```python
from build123d import *

# Parameters (mm, degrees)
EXTRUDE_THIN2_DEPTH = 25
SKETCH4_R           = 2.5
CUT_EXTRUDE1_DEPTH  = 0.3


with BuildPart() as part:
    # Sketch1 → Revolve1 (revolve)
    with BuildSketch(Plane.XY):
        Polygon((3.1, 16), (3.1, -16), (20, -16), (20, -12.5), (17, -12.5), (17, 12.5), (20, 12.5), (20, 16), align=None)
    revolve(axis=Axis((0, -1363.747655385, 0), (0, 1, 0)))

    # Sketch2 → Extrude-Thin2 (add)
    with BuildSketch(Plane(origin=(0, -12.5, 0), x_dir=(1, 0, 0), z_dir=(0, 1, 0))):
        with BuildLine():
            ThreePointArc((0, 17), (-17, 0), (0, -17))
            Line((0, -17), (89.2, -17))
            ThreePointArc((89.2, -17), (101.274072829, -7.735238064), (95.45, 6.325317547))
            Line((95.45, 6.325317547), (72.5003268, 19.575317547))
            Line((72.5003268, 19.575317547), (72.6503268, 19.835125168))
            Line((72.6503268, 19.835125168), (95.6, 6.585125168))
            ThreePointArc((95.6, 6.585125168), (101.563850577, -7.812883777), (89.2, -17.3))
            Line((89.2, -17.3), (0, -17.3))
            ThreePointArc((0, -17.3), (-17.3, 0), (0, 17.3))
            Line((0, 17.3), (0, 17))
        make_face()
    extrude(amount=EXTRUDE_THIN2_DEPTH)

    # Sketch4 → Cut-Extrude1 (cut)
    with BuildSketch(Plane(origin=(26.751442841, 0, -46.334858177), x_dir=(-0.866025404, 0, -0.5), z_dir=(0.5, 0, -0.866025404))):
        with Locations((-58.499466018, -7.5)):
            Circle(SKETCH4_R)
        with Locations((-58.499466018, 7.5)):
            Circle(SKETCH4_R)
    extrude(amount=-CUT_EXTRUDE1_DEPTH, mode=Mode.SUBTRACT)


solid = part.part
```
Input: part model. Units: mm. Frame: model coordinates. A direction names the side the tool comes from. Coordinates: 2 decimals unless noted, no trailing zeros. Order: outer loops, then holes, each group sorted by start corner. A loop starts at its lowest first (then second) coordinate and runs counter-clockwise, first axis right, second up. Notation, with made-up numbers: (-20, -7.5) - (12, -7.5) arc R28 cw to (12, 12.5) - close; hole circle Ø1 at (19.25, 57). An arc over 180 degrees is marked (long way). Return JSON: item names as keys, results as strings.
Q1. Cut plane B-B (z = -9.5). Return loops of the section in (x, y).
The answers:
{"outline": "(-17.6, -16) - (17.6, -16) - (17.6, -12.5) - (14.1, -12.5) - (14.1, 12.5) - (17.6, 12.5) - (17.6, 16) - (-17.6, 16) - (-17.6, 12.5) - (-14.46, 12.5) - (-14.46, -12.5) - (-17.6, -12.5) - close; (89.95, -12.5) - (90.55, -12.5) - (90.55, 12.5) - (89.95, 12.5) - close"}
Q2. Ray query, probe 1 along Y at (x, z) = (-6, 16.5); probe 2 along X at (y, z) = (1, 0); probe 3 along X at (y, z) = (4, 14). Return the intervals inside material, ascending.
The answers:
{"probe 1": "y = -16 to -12.5, 12.5 to 16", "probe 2": "x = -17.3 to -3.1, 3.1 to 17, 100.86 to 101.18", "probe 3": "x = -10.16 to 9.64, 97.32 to 97.78"}
Q3. Cut plane D-D (z = 14.5). Return loops of the section in (x, y).
The answers:
{"outline": "(-13.77, -16) - (13.77, -16) - (13.77, -12.5) - (8.87, -12.5) - (8.87, 12.5) - (13.77, 12.5) - (13.77, 16) - (-13.77, 16) - (-13.77, 12.5) - (-9.44, 12.5) - (-9.44, -12.5) - (-13.77, -12.5) - close; (96.7, -12.5) - (97.19, -12.5) - (97.19, 12.5) - (96.7, 12.5) - close"}
Q4. First-contact query: pin 1 (2 mm diameter, centred on x = -1, y = 0.5, fed in from +Z); pin 2 (1 mm diameter, centred on x = 11, y = 6.5, fed in from -Z); pin 3 (4 mm diameter, centred on x = 88.5, y = -11.5, fed in from -Z). Flat tips, straight axial feed; report the tip coordinate or a pass-through.
The answers:
{"pin 1": "stops at z = 17.3", "pin 2": "stops at z = -13.37", "pin 3": "stops at z = -11.84"}
Q5. Cut plane C-C (x = 43.5). Return loops of the section in (y, z).
The answers:
{"outline": "(-12.5, 17) - (12.5, 17) - (12.5, 17.3) - (-12.5, 17.3) - close"}
Q6. Cut plane A-A (z = 0). Return loops of the section in (x, y).
The answers:
{"outline": "(-20, -16) - (-3.1, -16) - (-3.1, 16) - (-20, 16) - (-20, 12.5) - (-17.3, 12.5) - (-17.3, -12.5) - (-20, -12.5) - close; (3.1, -16) - (20, -16) - (20, -12.5) - (17, -12.5) - (17, 12.5) - (20, 12.5) - (20, 16) - (3.1, 16) - close; (100.86, -12.5) - (101.18, -12.5) - (101.18, 12.5) - (100.86, 12.5) - close"}
Q7. Access query for faces 4 (the flat face through (9, 12.5, -15)), 5 (the cylindrical face through (-17.296, -0.175, 0.38)), 6 (the flat face through (84.136, -0.175, -12.858)). Directions: +Z, -Z, +X, -X, +Y, -Y. A direction counts if a zero-diameter tool reaches every point of the face in a straight line with its end or side. Return the directions, or none.
The answers:
{"face 4": "none", "face 5": "-X", "face 6": "+Y, -Y"}
Q8. Draft query along X for faces 1 (the cylindrical face through (17, 0, 0)), 2 (the cylindrical face through (-4.336, 14.274, 19.524)), 3 (the flat face through (45, 0, 17.3)). Return one class per face: +X half, -X half, draft (parallel to the pull), parting line (faces both ways), or undercut.
The answers:
{"face 1": "undercut", "face 2": "parting line", "face 3": "draft"}
